Could you check a few things on this model? Use its own coordinates, in mm. Give positions to 0.01 mm unless a question says otherwise; leave off trailing zeros. Write each loop counter-clockwise with the first axis right and the second up, starting at its lowest first coordinate (ties: lowest second). Pieces come first, ordered by that corner, then holes. Notation, with made-up numbers: (54.25, 54.5) - (84.25, 54.5) arc R13 ccw to (84.25, 79.5) - close; hole circle Ø11 at (46.5, 57.25). An arc over 180 degrees is marked (long way). Use one line per item in the form item = value.
```python
from build123d import *

# Parameters (mm, degrees)
F0_R     = 7.9375
F1_DEPTH = 12.7


with BuildPart() as f1:
    # F0 (on Top) → F1 (new body)
    with BuildSketch(Plane.XY):
        with BuildLine():
            ThreePointArc((31.8073335192, 20.9738774288), (37.4513031941, 7.0007063262), (37.2360288719, -8.0677229656))
            ThreePointArc((37.2360288719, -8.0677229656), (33.9725367984, -17.0138251575), (28.4983711579, -24.8059131627))
            Line((28.4983711579, -24.8059131627), (60.9339033423, 10.4515771637))
            ThreePointArc((60.9339033423, 10.4515771637), (40.4207699943, 13.0005062761), (49.4900105586, 31.5756120621))
            Line((49.4900105586, 31.5756120621), (33.9508555908, 28.9736107071))
            Line((33.9508555908, 28.9736107071), (31.8073335192, 20.9738774288))
        make_face()
        with BuildLine():
            ThreePointArc((49.4900105586, 31.5756120621), (40.4207699943, 13.0005062761), (60.9339033423, 10.4515771637))
            ThreePointArc((60.9339033423, 10.4515771637), (63.4193607937, 14.4353815135), (64.2874, 19.05))
            ThreePointArc((64.2874, 19.05), (59.79267739, 28.7434732141), (49.4900105586, 31.5756120621))
        make_face()
        with Locations((51.5874, 19.05)):
            Circle(F0_R, mode=Mode.SUBTRACT)
    extrude(amount=F1_DEPTH)


solid = f1.part
```
1. Imagine slicing it at B-B, the plane y = 17. List the corners of the cut face in (x, z) for me.
Response values:
outline = (34.1, 0) - (43.92, 0) - (43.92, 12.7) - (34.1, 12.7) - close; (59.26, 0) - (64.12, 0) - (64.12, 12.7) - (59.26, 12.7) - close
2. For pin 1 (1.5 mm diameter, centred on y = -8, z = 4, fed in from +X); pin 2 (6 mm diameter, centred on y = 9, z = 9, fed in from +X); pin 3 (1 mm diameter, centred on y = 12.5, z = 2.5, fed in from +X), each with a flat end and sliding along its axis, tell me the tip position at first contact or that it passes through.
Response values:
pin_1 = 44.65
pin_2 = 62.15
pin_3 = 62.75
3. If I drill on line 1 (X direction, y = 22, z = 3.25); line 2 (X direction, y = 26, z = 10.75); line 3 (Y direction, x = 58, z = 4.25), over which ranges is the centre line in solid material (lowest first)? Write a range as from..to.
Response values:
line_1 = 32.08..44.22, 58.96..63.94
line_2 = 33.15..47.75, 55.42..62.22
line_3 = 7.26..14.37, 23.73..30.01
4. Imagine slicing it at D-D, the plane x = 39. List the corners of the cut face in (y, z) for me.
Response values:
outline = (-13.39, 0) - (29.82, 0) - (29.82, 12.7) - (-13.39, 12.7) - close
5. Imagine slicing it at C-C, the plane x = 57.5. List the corners of the cut face in (y, z) for me, and give its area (3 significant figures).
Response values:
outline = (6.72, 0) - (13.75, 0) - (13.75, 12.7) - (6.72, 12.7) - close; (24.35, 0) - (30.29, 0) - (30.29, 12.7) - (24.35, 12.7) - close
area = 165 mm²
6. If we mould it in two halves opening along Y, with no side actions, what happens to faces 1 (the face through (46, 10, 12.7)), 2 (the face through (44.489, -7.424, 6.261)), 3 (the face through (37.41, 7.21, 6.26)), 4 (the face through (34.03, -16.9, 6.26))? For each: pulls with the +Y half, pulls with the -Y half, needs draft (parallel to the pull), parting line crosses it, or undercut.
Response values:
face_1 = needs draft
face_2 = pulls with the -Y half
face_3 = undercut
face_4 = undercut
